Answer from the drawing. Dimensions are ordinates in mm from the lowest x, y and z of the part. A direction names the side the tool comes from. Give positions to 0.01 mm unless a question says otherwise; leave off trailing zeros. Order: outer loops, then holes, each group sorted by start corner. A loop starts at its lowest first (then second) coordinate and runs counter-clockwise, first axis right, second up. Notation, with made-up numbers: M 21,51 L 60,51 A30 cw 60,87 Z; hole C -14.5,0 d7. An arc over 180 degrees is marked long. One line per item, written item: value.
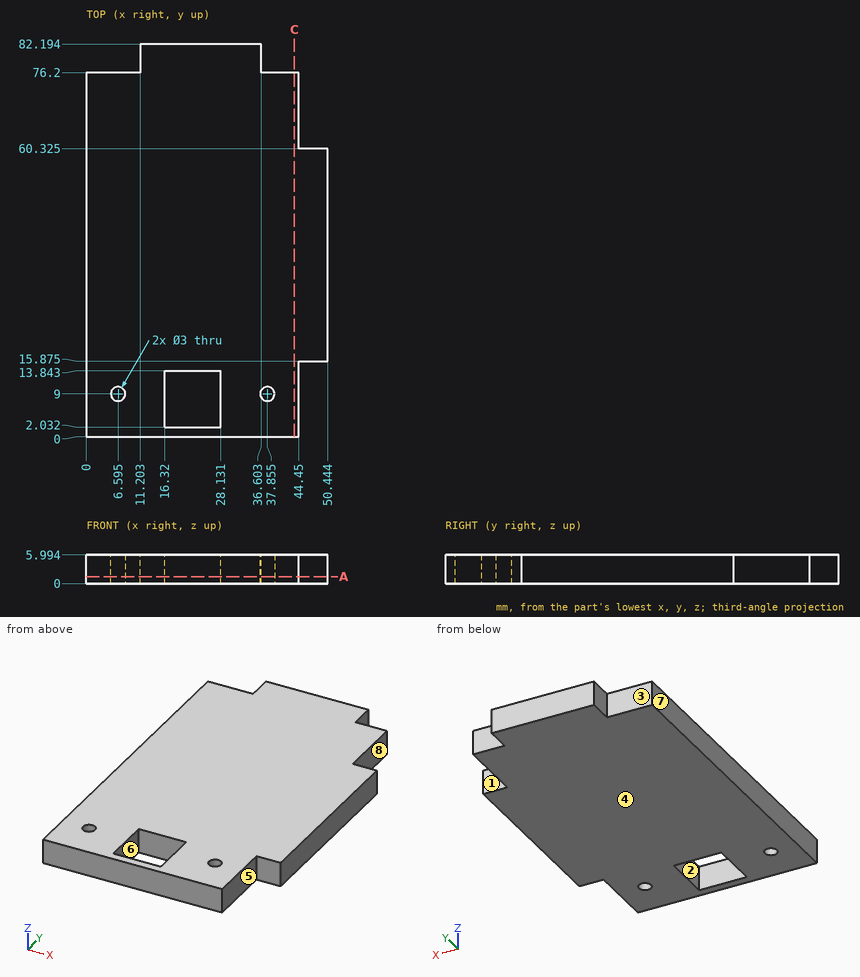
(1) Find the intervals of material crossed by probe 1 along Y at (x, z) = (16.5, 5.5) (1 decimal); probe 2 along X at (y, z) = (9.5, 0.75); probe 3 along Y at (x, z) = (11, 4.35), in increasing order. Write a range as from..to.
Findings:
probe 1: y = 0..2, 13.8..82.2
probe 2: x = 0..5.18, 8.01..16.32, 28.13..36.44, 39.27..44.45
probe 3: y = 0..76.2
(2) Section C-C, the plane x = 43.5 is taken. Give the vertices of the cut face in (y, z) (1 decimal), then the cut area to 3 significant figures.
Findings:
outline: M 0,0 L 76.2,0 L 76.2,6 L 0,6 Z
area: 457 mm^2
(3) Which of the six approach directions +Z, -Z, +X, -X, +Y, -Y give full straight-line access (tool end or side, diameter ignored) to the marked faces 1, 2, 3, 4 and 5?
Findings:
face 1: +Z, -Z, +X, +Y
face 2: +Z, -Z
face 3: +Z, -Z, -X, +Y
face 4: -Z, +X, -X, +Y, -Y
face 5: +Z, -Z, +X, -Y
(4) Given P1, Ø1.8, axis at y = 80, z = 4, coming from the -X side; P2, Ø1.8, axis at y = 8, z = 3.5, coming from the +X side; P3, Ø3, axis at x = 7, z = 3.5, coming from the +Y side, each flat-ended and moving along its own axis, determine where each tip first touches the part or whether it passes through.
Findings:
P1: stops at x = 11.2
P2: stops at x = 44.45
P3: stops at y = 76.2
(5) Section A-A, the plane z = 1.45 is taken. Give the number of separate pieces and of enclosed holes in the cut face, then the cut area to 3 significant figures.
Findings:
separate pieces: 1
enclosed holes: 3
area: 3,650 mm^2
(6) Determine the mould class of the marked faces 6, 7 and 8 for opening direction X: pulls with the +X half, pulls with the -X half, needs draft (parallel to the pull), parting line crosses it, or undercut.
Findings:
face 6: undercut
face 7: pulls with the -X half
face 8: pulls with the +X half
